The model under review builds one solid part; all positions refer to its coordinate system, in mm. Face numbers are marked on the shaded views. Round coordinates to 2 decimals unless told otherwise and drop trailing zeros. Loops run counter-clockwise (first coordinate to the right, second up) from the corner with the lowest first, then second, coordinate; pieces in that order, holes last. Notation, with made-up numbers: (0, 66) -> (38, 66) arc R21 ccw to (38, 90) -> close; hole circle Ø5 at (-30, 18.5). An arc over 180 degrees is marked (long way). Use a Markdown table: item, result. Add a question column.
1) Consider section B-B on x = -30.5. Give the boundary of the cut face in (y, z), plus the area to 3 significant figures.
2) Insertion check: pin 1 (3 mm diameter, centred on x = 20, z = 10, fed in from -Y); pin 2 (8 mm diameter, centred on x = -36, z = 33, fed in from +Y); pin 3 (3 mm diameter, centred on y = -31, z = 27, fed in from -X). Each pin has a flat end and moves straight along its axis. Give the tip position at first contact, or say it passes through.
3) Mouldability with a two-part tool opening along Z and no side actions: class the marked faces 1, 2 and 3 as released by +Z, released by -Z, zero draft, split by the parting line, or undercut.
4) Consider section C-C on y = 42. Give the boundary of the cut face in (x, z).
5) Consider section D-D on z = -11.5. Give the boundary of the cut face in (x, y), plus the area to 3 significant figures.
6) Wall thickness on probe 1 along Z at (x, y) = (44.5, -6); probe 2 along Z at (x, y) = (-38.5, 26.5); probe 3 along Z at (x, y) = (14.5, -14): over which ranges is each line inside the solid? List them lowest first.
7) Consider section A-A on y = 0. Give the boundary of the cut face in (x, z), plus the area to 3 significant figures.
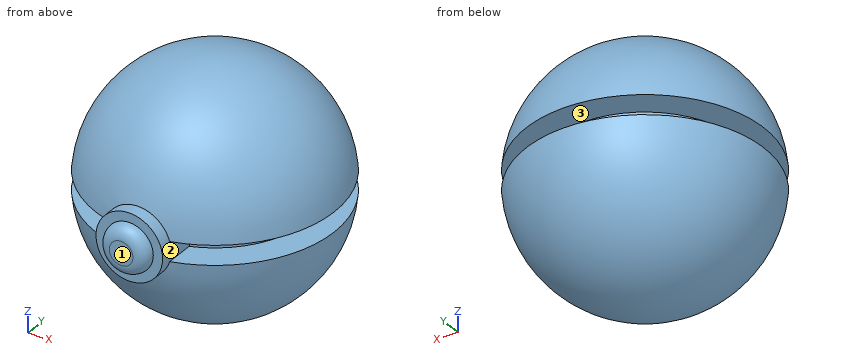
from build123d import *

# Parameters (mm, degrees)
F2_R     = 13.922185385
F3_DEPTH = 53.34
F4_R     = 10.0272817178
F5_DEPTH = 5.08
F6_R     = 5.07999


# Not quite as in the source:
# - a fillet or chamfer is up to 0.001 mm smaller than in the source, because OpenCascade refuses the exact size


with BuildPart() as f1:
    # F0 (on Front) → F1 (revolve)
    with BuildSketch(Plane.XZ):
        with BuildLine():
            Line((0, 0), (0, -50))
            ThreePointArc((0, -50), (33.8768500277, -36.7744344919), (49.8320800855, -4.0943612879))
            Line((49.8320800855, -4.0943612879), (38.2781662047, -4.0943612879))
            Line((38.2781662047, -4.0943612879), (38.2781662047, 0))
            Line((38.2781662047, 0), (38.2781662047, 4.0943612879))
            Line((38.2781662047, 4.0943612879), (49.8320800855, 4.0943612879))
            ThreePointArc((49.8320800855, 4.0943612879), (33.8768500277, 36.7744344919), (0, 50))
            Line((0, 50), (0, 0))
        make_face()
    revolve(axis=Axis((0, 0, 25), (0, 0, 1)))

    # F2 (on Front) → F3 (join)
    with BuildSketch(Plane.XZ):
        Circle(F2_R)
    extrude(amount=F3_DEPTH)

    # F4 (on face) → F5 (join)
    with BuildSketch(Plane.XZ.offset(53.34)):
        Circle(F4_R)
    extrude(amount=F5_DEPTH)

    # F6 (radius 5.08 in the source; OpenCascade refuses exactly that, so slightly less here)
    f6_edges = [f1.edges().sort_by_distance(p)[0] for p in [
        (-10.027282, -58.42, 0),
    ]]
    fillet(f6_edges, radius=F6_R)


solid = f1.part
Result set:
| question | item | result |
|---|---|---|
| 1 | outline | (-39.41, -4.09) arc R39.62 ccw to (39.41, -4.09) -> (23.13, -4.09) -> (23.13, 4.09) -> (39.41, 4.09) arc R39.62 ccw to (-39.41, 4.09) -> (-23.13, 4.09) -> (-23.13, -4.09) -> close |
| 1 | area | 4,660 mm2 |
| 2 | pin 1 | y = -45.44 |
| 2 | pin 2 | y = 22.13 |
| 2 | pin 3 | x = -30.51 |
| 3 | face 1 | zero draft |
| 3 | face 2 | undercut |
| 3 | face 3 | undercut |
| 4 | outline | (-26.82, -4.09) arc R27.13 ccw to (26.82, -4.09) -> close; (-26.82, 4.09) -> (26.82, 4.09) arc R27.13 ccw to start |
| 5 | outline | (-7.85, -53.34) -> (7.85, -53.34) -> (7.85, -48.02) arc R48.66 ccw (long way) to (-7.85, -48.02) -> close |
| 5 | area | 7,520 mm2 |
| 6 | probe 1 | -21.99 to -4.09, 4.09 to 21.99 |
| 6 | probe 2 | -17.76 to -4.09, 4.09 to 17.76 |
| 6 | probe 3 | -45.76 to 45.76 |
| 7 | outline | (-49.83, -4.09) arc R50 ccw to (49.83, -4.09) -> (38.28, -4.09) -> (38.28, 4.09) -> (49.83, 4.09) arc R50 ccw to (-49.83, 4.09) -> (-38.28, 4.09) -> (-38.28, -4.09) -> close |
| 7 | area | 7,660 mm2 |
